Read the model definition and answer for the solid it produces. Units are mm, in the model's axes. Give positions to 0.01 mm unless a question says otherwise; leave off trailing zeros. Order: outer loops, then holes, each group sorted by start corner. A loop starts at its lowest first (then second) coordinate and runs counter-clockwise, first axis right, second up. Notation, with made-up numbers: (39.25, 81.5) - (88.25, 81.5) arc R15 ccw to (88.25, 103.5) - close; hole circle Ø11 at (-24.75, 78.25). An arc over 180 degrees is marked (long way). Return JSON: item names as keys, results as strings.
```python
from build123d import *

# Parameters (mm, degrees)
SKETCH1_W           = 140
SKETCH1_H           = 81.5
BOSS_EXTRUDE1_DEPTH = 10
SKETCH2_R           = 14
CUT_EXTRUDE2_DEPTH  = 8
SKETCH5_R           = 5
SKETCH5_R_2         = 2.6
SKETCH5_R_3         = 3.1
CUT_EXTRUDE4_DEPTH  = 82.612269298
SKETCH25_W          = 35
SKETCH25_H          = 5
CUT_EXTRUDE6_DEPTH  = 82.612269298
CHAMFER2_SIZE       = 10
SKETCH27_R          = 10
CUT_EXTRUDE8_DEPTH  = 3
CIRPATTERN1_COUNT   = 4


with BuildPart() as part:
    # Sketch1 → Boss-Extrude1 (new body)
    with BuildSketch(Plane.XY):
        Rectangle(SKETCH1_W, SKETCH1_H)
    extrude(amount=BOSS_EXTRUDE1_DEPTH)

    # Sketch2 → Cut-Extrude2 (cut)
    with BuildSketch(Plane(origin=(0, 0, 0), x_dir=(-1, 0, 0), z_dir=(0, 0, -1))):
        with Locations((0, 9.25)):
            Circle(SKETCH2_R)
    extrude(amount=-CUT_EXTRUDE2_DEPTH, mode=Mode.SUBTRACT)

    # Sketch5 → Cut-Extrude4 (cut, through all)
    with BuildSketch(Plane(origin=(0, 0, 0), x_dir=(-1, 0, 0), z_dir=(0, 0, -1))):
        with Locations((-60, 19.25)):
            Circle(SKETCH5_R)
        with Locations((60, 19.25)):
            Circle(SKETCH5_R)
        with Locations((-60, 35.25)):
            Circle(SKETCH5_R_2)
        with Locations((-60, 3.25)):
            Circle(SKETCH5_R_2)
        with Locations((60, 35.25)):
            Circle(SKETCH5_R_2)
        with Locations((60, 3.25)):
            Circle(SKETCH5_R_2)
        with Locations((-60, -30.75)):
            Circle(SKETCH5_R_3)
        with Locations((-40, -30.75)):
            Circle(SKETCH5_R_3)
        with Locations((40, -30.75)):
            Circle(SKETCH5_R_3)
        with Locations((60, -30.75)):
            Circle(SKETCH5_R_3)
    extrude(amount=-CUT_EXTRUDE4_DEPTH, mode=Mode.SUBTRACT)

    # Sketch25 → Cut-Extrude6 (cut, through all)
    with BuildSketch(Plane.XY.offset(10)):
        with Locations((0, -38.25)):
            Rectangle(SKETCH25_W, SKETCH25_H)
    extrude(amount=-CUT_EXTRUDE6_DEPTH, mode=Mode.SUBTRACT)

    # Chamfer2
    # the kernel refuses this chamfer: 10 mm, written as the material it adds along each edge
    with BuildSketch(Plane(origin=(17.5, -35.75, 10), x_dir=(-0.9996219169112968, 0.027495876610586317, 0), z_dir=(0, 0, -1))) as chamfer2_piece_1_section:
        Polygon((CHAMFER2_SIZE * 0.999621916911, -CHAMFER2_SIZE * 0.0274958766106), (-CHAMFER2_SIZE * 0.0274958766106, -CHAMFER2_SIZE * 0.999621916911), (0, 0), align=None)
    chamfer2_piece_1 = extrude(amount=10, mode=Mode.PRIVATE)
    chamfer2_piece_1 = split(chamfer2_piece_1, bisect_by=Plane(origin=(13.565989159, -40.75, 5), z_dir=(0, 1, 0)), keep=Keep.TOP, mode=Mode.PRIVATE)
    add(chamfer2_piece_1)
    with BuildSketch(Plane(origin=(-17.5, -35.75, 10), x_dir=(-0.027495876610586317, -0.9996219169112968, 0), z_dir=(0, 0, -1))) as chamfer2_piece_2_section:
        Polygon((CHAMFER2_SIZE * 0.999621916911, -CHAMFER2_SIZE * 0.0274958766106), (-CHAMFER2_SIZE * 0.0274958766106, -CHAMFER2_SIZE * 0.999621916911), (0, 0), align=None)
    chamfer2_piece_2 = extrude(amount=10, mode=Mode.PRIVATE)
    chamfer2_piece_2 = split(chamfer2_piece_2, bisect_by=Plane(origin=(-13.565989159, -40.75, 5), z_dir=(0, 1, 0)), keep=Keep.TOP, mode=Mode.PRIVATE)
    add(chamfer2_piece_2)

    # Sketch27 → Cut-Extrude8 (cut)
    with BuildSketch(Plane(origin=(0, 0, 8), x_dir=(-1, 0, 0), z_dir=(0, 0, -1))):
        with Locations((0, 9.25)):
            Circle(SKETCH27_R)
    extrude(amount=-CUT_EXTRUDE8_DEPTH, mode=Mode.SUBTRACT)

    # Sketch30 → M4 Tapped Hole1 (revolve, cut)
    with BuildSketch(Plane(origin=(0, 27.25, 0), x_dir=(0, 1, 0), z_dir=(1, 0, 0))):
        Polygon((0, 0), (0, 11.091420021), (1.65, 10.1), (1.65, 0), align=None)
    m4_tapped_hole1 = revolve(axis=Axis((0, 27.25, -6.35), (0, 0, 1)), mode=Mode.SUBTRACT)

    # CirPattern1: M4 Tapped Hole1 ×4 about axis
    cirpattern1_axis = Axis((0, 9.25, 0), (0, 0, 1))
    for i in range(1, CIRPATTERN1_COUNT):
        add(m4_tapped_hole1.rotate(cirpattern1_axis, i * 360 / CIRPATTERN1_COUNT), mode=Mode.SUBTRACT)


solid = part.part
```
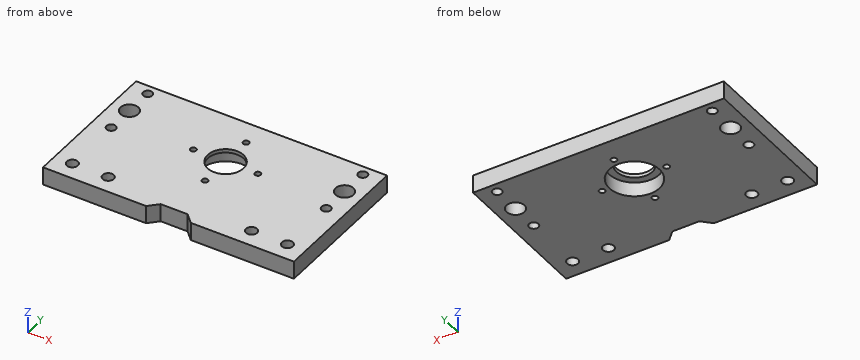
Q1. Given pin 1 (22.5 mm diameter, centred on x = 2, y = 8.5, fed in from -Z), flat-ended and moving along its own axis, determine where the tip first touches the part or whether it passes through.
Values:
{"pin 1": "stops at z = 8"}
Q2. Consider L1, parallel to Y at x = 60, z = 6; L2, parallel to X at y = 35.5, z = 7.75; L3, parallel to X at y = 27.25, z = 2.75. Determine where each line is inside the solid, lowest interval first.
Values:
{"L1": "y = -40.75 to -33.85, -27.65 to 0.65, 5.85 to 14.25, 24.25 to 32.65, 37.85 to 40.75", "L2": "x = -70 to -62.59, -57.41 to 57.41, 62.59 to 70", "L3": "x = -70 to -1.65, 1.65 to 70"}
Q3. A cutting plane is placed at D-D (z = 1.5). Give the number of separate pieces and of enclosed holes in the cut face, and give its area (3 significant figures).
Values:
{"separate pieces": "1", "enclosed holes": "15", "area": "10,300 mm²"}
Q4. A cutting plane is placed at C-C (x = -40). Write down the section's boundary in (y, z), and give its area (3 significant figures).
Values:
{"outline": "(-40.75, 0) - (-33.85, 0) - (-33.85, 10) - (-40.75, 10) - close; (-27.65, 0) - (40.75, 0) - (40.75, 10) - (-27.65, 10) - close", "area": "753 mm²"}
Q5. A cutting plane is placed at B-B (y = -30.75). Write down the section's boundary in (x, z).
Values:
{"outline": "(-70, 0) - (-63.1, 0) - (-63.1, 10) - (-70, 10) - close; (-56.9, 0) - (-43.1, 0) - (-43.1, 10) - (-56.9, 10) - close; (-36.9, 0) - (36.9, 0) - (36.9, 10) - (-36.9, 10) - close; (43.1, 0) - (56.9, 0) - (56.9, 10) - (43.1, 10) - close; (63.1, 0) - (70, 0) - (70, 10) - (63.1, 10) - close"}
Q6. A cutting plane is placed at A-A (x = 0). Write down the section's boundary in (y, z).
Values:
{"outline": "(-35.75, 0) - (-10.4, 0) - (-10.4, 10) - (-35.75, 10) - close; (-7.1, 0) - (-4.75, 0) - (-4.75, 8) - (-0.75, 8) - (-0.75, 10) - (-7.1, 10) - close; (19.25, 8) - (23.25, 8) - (23.25, 0) - (25.6, 0) - (25.6, 10) - (19.25, 10) - close; (28.9, 0) - (40.75, 0) - (40.75, 10) - (28.9, 10) - close"}
